```python
from build123d import *

# Parameters (mm, degrees)
SKETCH3_R           = 2.4892
BOSS_EXTRUDE1_DEPTH = 3.175


with BuildPart() as part:
    # Sketch3 → Boss-Extrude1 (new body)
    with BuildSketch(Plane(origin=(0, 0, 0), x_dir=(0, 0, -1), z_dir=(1, 0, 0))):
        Polygon((0, 0), (38.1, 0), (38.1, 12.7), (12.7, 50.8), (0, 50.8), align=None)
        with Locations((6.35, 44.45)):
            Circle(SKETCH3_R, mode=Mode.SUBTRACT)
        with Locations((6.35, 31.75)):
            Circle(SKETCH3_R, mode=Mode.SUBTRACT)
        with Locations((6.35, 6.35)):
            Circle(SKETCH3_R, mode=Mode.SUBTRACT)
        with Locations((31.75, 6.35)):
            Circle(SKETCH3_R, mode=Mode.SUBTRACT)
    extrude(amount=BOSS_EXTRUDE1_DEPTH)


solid = part.part
```
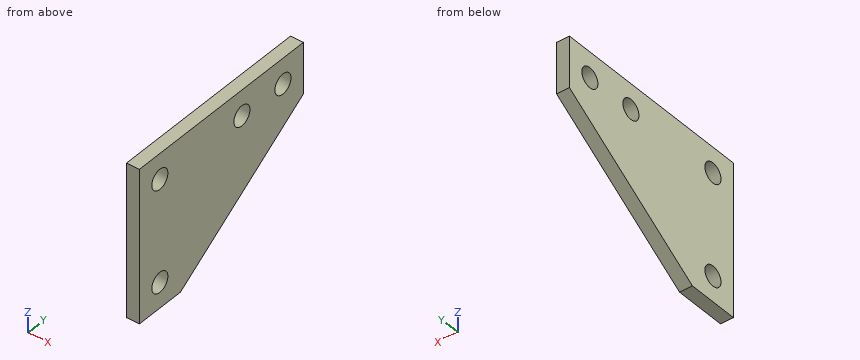
Read the model definition and answer for the solid it produces. Units are mm, in the model's axes. Coordinates: 2 decimals unless noted, no trailing zeros. Write each loop counter-clockwise with the first axis right and the second up, starting at its lowest first coordinate (ties: lowest second). Pieces come first, ordered by that corner, then holes. Notation, with made-up numbers: (76.5, 34) -> (134.5, 34) arc R31 cw to (134.5, 66) -> close; hole circle Ø2 at (85.5, -35). An arc over 180 degrees is marked (long way). Answer as a JSON object with one key per item and string values.
Q1. A flat-ended cylindrical pin translates along its axis: pin 1 Ø4.5 at (y, z) = (31.75, -6.35) entering from +X. Find the tip coordinate at first contact, or state that the pin passes through.
The answers:
{"pin 1": "passes through"}
Q2. The part is cut by section D-D on y = 31.75. Give the vertices of the cut face in (x, z) (3 decimals), then the cut area to 3 significant figures.
The answers:
{"outline": "(0, -25.4) -> (3.175, -25.4) -> (3.175, -8.839) -> (0, -8.839) -> close; (0, -3.861) -> (3.175, -3.861) -> (3.175, 0) -> (0, 0) -> close", "area": "64.8 mm2"}
Q3. Consider line 1 (Y direction, x = 1.7, z = -6.35); line 2 (Z direction, x = 2.9, y = 6); line 3 (Z direction, x = 1.1, y = 44.5). Determine where each line is inside the solid, lowest interval first. Write a range as [from, to].
The answers:
{"line 1": "y = [0, 3.86], [8.84, 29.26], [34.24, 41.96], [46.94, 50.8]", "line 2": "z = [-38.1, -34.21], [-29.29, -8.81], [-3.89, 0]", "line 3": "z = [-16.9, -8.84], [-3.86, 0]"}
Q4. The part is cut by section A-A on z = -6.35. Give the vertices of the cut face in (x, y) (3 decimals).
The answers:
{"outline": "(0, 0) -> (3.175, 0) -> (3.175, 3.861) -> (0, 3.861) -> close; (0, 8.839) -> (3.175, 8.839) -> (3.175, 29.261) -> (0, 29.261) -> close; (0, 34.239) -> (3.175, 34.239) -> (3.175, 41.961) -> (0, 41.961) -> close; (0, 46.939) -> (3.175, 46.939) -> (3.175, 50.8) -> (0, 50.8) -> close"}
Q5. The part is cut by section B-B on y = 6.35. Give the vertices of the cut face in (x, z) (3 decimals).
The answers:
{"outline": "(0, -38.1) -> (3.175, -38.1) -> (3.175, -34.239) -> (0, -34.239) -> close; (0, -29.261) -> (3.175, -29.261) -> (3.175, -8.839) -> (0, -8.839) -> close; (0, -3.861) -> (3.175, -3.861) -> (3.175, 0) -> (0, 0) -> close"}
Q6. The part is cut by section C-C on x = 1.1. Give the vertices of the cut face in (y, z).
The answers:
{"outline": "(0, -38.1) -> (12.7, -38.1) -> (50.8, -12.7) -> (50.8, 0) -> (0, 0) -> close; hole circle Ø4.98 at (6.35, -31.75); hole circle Ø4.98 at (6.35, -6.35); hole circle Ø4.98 at (31.75, -6.35); hole circle Ø4.98 at (44.45, -6.35)"}
